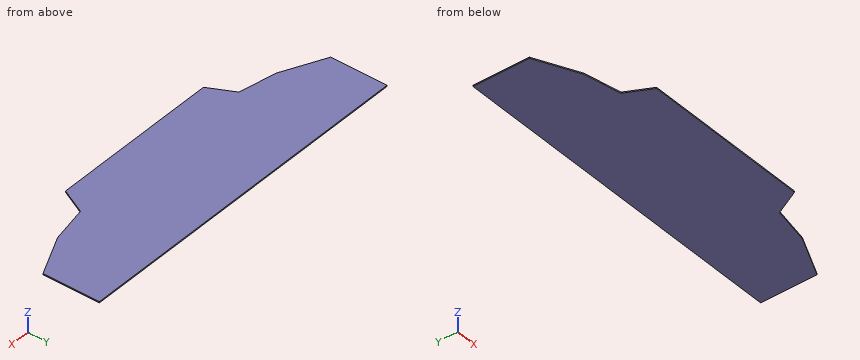
from build123d import *

# Parameters (mm, degrees)
F1_DEPTH = 6.35


with BuildPart() as f1:
    # F0 (on Top) → F1 (new body)
    with BuildSketch(Plane.XY):
        Polygon((-525.438485, -16.130894), (-457.2, -152.4), (0, -152.4), (0, 435.37514), (-953.46813, 435.37514), (-953.46813, 130.57514), (-724.837154, 22.989569), align=None)
    extrude(amount=F1_DEPTH)

    # F2: F1 across plane


with BuildPart() as f1_1:
    add(f1.part)
    add(f1.part.mirror(Plane.YZ))


solid = f1_1.part
Input: part model. Units: mm. Frame: model coordinates. Coordinates: 2 decimals unless noted, no trailing zeros. Loops run counter-clockwise (first coordinate to the right, second up) from the corner with the lowest first, then second, coordinate; pieces in that order, holes last. Notation, with made-up numbers: (-5.75, 56) -> (13.25, 56) arc R32 cw to (13.25, 90) -> close; hole circle Ø3 at (-29, -37). An arc over 180 degrees is marked (long way). Write each question's results on one line, items separated by ' | '. Start each with the question number.
Q1. Ray query, line 1 (X direction, y = -81, z = 0.75); line 2 (Y direction, x = 812, z = 3.5); line 3 (X direction, y = 107.5, z = 2). Return the intervals inside material, ascending. Write a range as from..to.
Q2. Section A-A, the plane z = 3.25. Return the cut outline in (x, y).
Q3. Section B-B, the plane y = 59.5. Return the cut outline in (x, z).
Q4. Section C-C, the plane x = 705. Return the cut outline in (y, z).
Found:
1) line 1: -492.95..492.95 | line 2: 64.01..435.38 | line 3: -904.43..904.43
2) outline: (-953.47, 130.58) -> (-724.84, 22.99) -> (-525.44, -16.13) -> (-457.2, -152.4) -> (457.2, -152.4) -> (525.44, -16.13) -> (724.84, 22.99) -> (953.47, 130.58) -> (953.47, 435.38) -> (-953.47, 435.38) -> close
3) outline: (-802.43, 0) -> (802.43, 0) -> (802.43, 6.35) -> (-802.43, 6.35) -> close
4) outline: (19.1, 0) -> (435.38, 0) -> (435.38, 6.35) -> (19.1, 6.35) -> close
